CAD build for the part. Positions are in the model's coordinates, mm. A direction names the side the tool comes from. Coordinates: 2 decimals unless noted, no trailing zeros. Order: outer loops, then holes, each group sorted by start corner. A loop starts at its lowest first (then second) coordinate and runs counter-clockwise, first axis right, second up. Notation, with made-up numbers: (53, 7) -> (89, 7) arc R22 cw to (89, 39) -> close; hole circle Ø4 at (-22.75, 42.25). An arc over 180 degrees is marked (long way). Use one line per item in the form item = value. Start each with the question number.
from build123d import *

# Parameters (mm, degrees)
SKETCH1_W           = 7
SKETCH1_H           = 15
SKETCH1_W_2         = 8
BOSS_EXTRUDE1_DEPTH = 2
SKETCH2_W           = 8
SKETCH2_H           = 15
BOSS_EXTRUDE2_DEPTH = 2
SKETCH3_W           = 8
SKETCH3_H           = 15
BOSS_EXTRUDE4_DEPTH = 2
SKETCH4_R           = 1.665
SKETCH4_R_2         = 1.65
CUT_EXTRUDE1_DEPTH  = 9
FILLET1_R           = 2.1
FILLET2_R           = 2.1
SKETCH5_W           = 12
SKETCH5_H           = 3
CUT_EXTRUDE2_DEPTH  = 3.8
SKETCH6_R           = 1.5
CUT_EXTRUDE3_DEPTH  = 17.2
FILLET3_R           = 1
FILLET4_R           = 1
SKETCH7_W           = 12
SKETCH7_H           = 3
CUT_EXTRUDE4_DEPTH  = 0.2


with BuildPart() as part:
    # Sketch1 → Boss-Extrude1 (new body)
    with BuildSketch(Plane(origin=(0, 0, 0), x_dir=(1, 0, 0), z_dir=(0, 1, 0))):
        with Locations((-3.5, 7.5)):
            Rectangle(SKETCH1_W, SKETCH1_H)
        with Locations((4, 7.5)):
            Rectangle(SKETCH1_W_2, SKETCH1_H)
    extrude(amount=BOSS_EXTRUDE1_DEPTH)

    # Sketch2 → Boss-Extrude2 (add)
    with BuildSketch(Plane.XZ):
        with Locations((-3, -7.5)):
            Rectangle(SKETCH2_W, SKETCH2_H)
    extrude(amount=BOSS_EXTRUDE2_DEPTH)

    # Sketch3 → Boss-Extrude4 (add)
    with BuildSketch(Plane(origin=(0, 2, 0), x_dir=(1, 0, 0), z_dir=(0, 1, 0))):
        with Locations((-3, 7.5)):
            Rectangle(SKETCH3_W, SKETCH3_H)
    extrude(amount=BOSS_EXTRUDE4_DEPTH)

    # Sketch4 → Cut-Extrude1 (cut)
    with BuildSketch(Plane(origin=(0, 0, 0), x_dir=(-1, 0, 0), z_dir=(0, -1, 0))):
        with Locations((-4.5, 3.75)):
            Circle(SKETCH4_R)
        with Locations((-4.5, 11.25)):
            Circle(SKETCH4_R_2)
    extrude(amount=-CUT_EXTRUDE1_DEPTH, mode=Mode.SUBTRACT)

    # Fillet1
    fillet1_edges = [part.edges().sort_by_distance(p)[0] for p in [
        (8, 1, 0),
    ]]
    fillet(fillet1_edges, radius=FILLET1_R)

    # Fillet2
    fillet2_edges = [part.edges().sort_by_distance(p)[0] for p in [
        (8, 1, -15),
    ]]
    fillet(fillet2_edges, radius=FILLET2_R)

    # Sketch5 → Cut-Extrude2 (cut)
    with BuildSketch(Plane.ZY.offset(7)):
        with Locations((-7.5, 0.736813471)):
            Rectangle(SKETCH5_W, SKETCH5_H)
    extrude(amount=-CUT_EXTRUDE2_DEPTH, mode=Mode.SUBTRACT)

    # Sketch6 → Cut-Extrude3 (cut)
    with BuildSketch(Plane(origin=(0, 4, 0), x_dir=(1, 0, 0), z_dir=(0, 1, 0))):
        with Locations((-5, 7.5)):
            Circle(SKETCH6_R)
    extrude(amount=-CUT_EXTRUDE3_DEPTH, mode=Mode.SUBTRACT)

    # Fillet3
    fillet3_edges = [part.edges().sort_by_distance(p)[0] for p in [
        (1, 0, -7.5),
    ]]
    fillet(fillet3_edges, radius=FILLET3_R)

    # Fillet4
    fillet4_edges = [part.edges().sort_by_distance(p)[0] for p in [
        (1, 2, -7.5),
    ]]
    fillet(fillet4_edges, radius=FILLET4_R)

    # Sketch7 → Cut-Extrude4 (cut)
    with BuildSketch(Plane.ZY.offset(3.2)):
        with Locations((-7.5, 0.736813471)):
            Rectangle(SKETCH7_W, SKETCH7_H)
    extrude(amount=-CUT_EXTRUDE4_DEPTH, mode=Mode.SUBTRACT)


solid = part.part
1) Cut at A-A on z = -3.75. Give the cut face in (x, y) (3 decimals), then the cut area to 3 significant figures.
2) Two-plate mould, pull along Y, no slides. Class faces 4 (the face through (1.301, -0.285, -7.395)), 5 (the face through (-5, 1, -1.5)), 6 (the face through (-2, 1, -15)), 7 (the face through (-5, 1, -13.5)): released by +Y, released by -Y, zero draft, split by the parting line, or undercut.
3) Probe L1, parallel to X at y = -1.25, z = -7.5; L2, parallel to X at y = 1.55, z = -3.75 (3 decimals); L3, parallel to Z at x = 4.5, y = 0.8 (3 decimals). List the from-to ranges inside material, lowest first.
4) Cut at C-C on y = 0.9. Give the cut face in (x, z) (3 decimals).
5) Cut at B-B on x = -5. Give the cut face in (y, z), then the cut area to 3 significant figures.
6) Cut at D-D on z = -7.5. Give the cut face in (x, y).
7) 3-axis set-ups, long thin cutter, end or side, ignore diameter. For faces 1 (the face through (-6, 2.237, -9)), 2 (the face through (8, 1, -7)), 3 (the face through (1, -1.5, -7.6)): which of +Z, -Z, +X, -X, +Y, -Y reach the whole face in a straight line?
8) Drop flat-ended pins along their axis: P1, Ø3, axis at x = 4.5, z = -11, coming from the +Y side; P2, Ø0.8, axis at y = 3.5, z = -8, coming from the +X side; P3, Ø5, axis at x = 4.5, z = -7.5, coming from the -Y side; P4, Ø1.5, axis at x = -5.5, y = 0.5, coming from the +Z side. Give the stop position or say it passes through.
Values follow:
q1.outline = (-7, -2) -> (1, -2) -> (1, -1) arc R1 cw to (2, 0) -> (2.835, 0) -> (2.835, 2) -> (2, 2) arc R1 cw to (1, 3) -> (1, 4) -> (-7, 4) -> (-7, 2.237) -> (-3, 2.237) -> (-3, -0.763) -> (-7, -0.763) -> close; (6.165, 0) -> (8, 0) -> (8, 2) -> (6.165, 2) -> close
q1.area = 43.8 mm^2
q2.face_4 = released by -Y
q2.face_5 = undercut
q2.face_6 = zero draft
q2.face_7 = undercut
q3.L1 = -7 to -6.5, -3.5 to 1
q3.L2 = -3 to 2.835, 6.165 to 8
q3.L3 = -15 to -12.9, -9.6 to -5.415, -2.085 to 0
q4.outline = (-7, -15) -> (5.9, -15) arc R2.1 ccw to (8, -12.9) -> (8, -2.1) arc R2.1 ccw to (5.9, 0) -> (-7, 0) -> (-7, -1.5) -> (-3, -1.5) -> (-3, -13.5) -> (-7, -13.5) -> close; hole circle Ø3.33 at (4.5, -3.75); hole circle Ø3.3 at (4.5, -11.25)
q5.outline = (-2, -15) -> (4, -15) -> (4, -9) -> (2.24, -9) -> (2.24, -13.5) -> (-0.76, -13.5) -> (-0.76, -9) -> (-2, -9) -> close; (-2, -6) -> (-0.76, -6) -> (-0.76, -1.5) -> (2.24, -1.5) -> (2.24, -6) -> (4, -6) -> (4, 0) -> (-2, 0) -> close
q5.area = 45.0 mm^2
q6.outline = (-7, -2) -> (-6.5, -2) -> (-6.5, -0.76) -> (-7, -0.76) -> close; (-7, 2.24) -> (-6.5, 2.24) -> (-6.5, 4) -> (-7, 4) -> close; (-3.5, -2) -> (1, -2) -> (1, -1) arc R1 cw to (2, 0) -> (8, 0) -> (8, 2) -> (2, 2) arc R1 cw to (1, 3) -> (1, 4) -> (-3.5, 4) -> (-3.5, 2.24) -> (-3, 2.24) -> (-3, -0.76) -> (-3.5, -0.76) -> close
q7.face_1 = -X
q7.face_2 = +Z, -Z, +X, +Y, -Y
q7.face_3 = +Z, -Z, +X, -Y
q8.P1 = 2
q8.P2 = 1
q8.P3 = 0
q8.P4 = 0
